Part model, mm, in its own coordinate system. A direction names the side the tool comes from. Give positions to 0.01 mm unless a question says otherwise; leave off trailing zeros. Order: outer loops, then holes, each group sorted by start corner. A loop starts at its lowest first (then second) coordinate and runs counter-clockwise, first axis right, second up.
1. Probe line 1 (X direction, y = -17.25, z = 0); line 2 (Z direction, x = -14.5, y = -19.25); line 3 (Z direction, x = -17, y = -25). List the from-to ranges inside material, lowest first.
2. Slice it at C-C on y = -12.5. List the corners of the cut face in (x, z).
3. Which spindle directions (+Z, -Z, +X, -X, +Y, -Y) get a long thin tool onto all of the face, cutting with end or side? Do faces 4 (the cylindrical face through (-19.62, -15.42, 2.95)), 5 (the flat face through (-14, -8.753, 4)). Say none if no direction does.
4. Mould opens along Y. For faces 1 (the cylindrical face through (-17.355, -15.705, 5.207)), 2 (the flat face through (-20, -21.753, 1)), 3 (the flat face through (-18, -33.753, -3)) say: +Y half, -Y half, draft (parallel to the pull), parting line (faces both ways), or undercut.
5. Drop flat-ended pins along their axis: pin 1 Ø2 at (x, z) = (-20, 0) entering from +Y; pin 2 Ø4 at (x, y) = (-20.5, -15) entering from +Z; pin 3 Ø4 at (x, y) = (-12, -12) entering from +Z; pin 4 Ø5 at (x, y) = (-16.92, -28.75) entering from +Z. Give the stop position or say it passes through.
6. Slice it at D-D on y = -16.25. List the corners of the cut face in (x, z).
7. Slice it at A-A on y = -30. List the corners of the cut face in (x, z).
8. Slice it at B-B on x = -15.25. Give the number of separate pieces and of enclosed holes in the cut face, and give its area (3 significant figures).
from build123d import *

# Parameters (mm, degrees)
WYTNIJ_WYCI_GNI_CIE1_DEPTH      = 42.958230131
WYTNIJ_WYCI_GNI_CIE1_DEPTH_BACK = 42.958230131
SZKIC2_R                        = 2
SFAZOWANIE1_SIZE                = 0.5
ZAOKR_GLENIE1_R                 = 0.5
SFAZOWANIE2_SIZE                = 0.5


with BuildPart() as part:
    # Szkic1 → Obrót1 (revolve)
    with BuildSketch(Plane.XY, mode=Mode.PRIVATE) as obr_t1_sk:
        Polygon((-20.921239747, -8.753034896), (-23.921239747, -8.753034896), (-23.921239747, -33.753034896), (-19.421239747, -33.753034896), (-19.421239747, -21.753034896), (-20.921239747, -21.753034896), align=None)
    revolve(obr_t1_sk.sketch.rotate(Axis((-16.921239747, -33.753034896, 0), (0, 1, 0)), 270), axis=Axis((-16.921239747, -33.753034896, 0), (0, 1, 0)))

    # Szkic2 → Wytnij-wyciągnięcie1 (cut, two sides: drawn at the far end of the back side and taken through both)
    with BuildSketch(Plane.XY.offset(-WYTNIJ_WYCI_GNI_CIE1_DEPTH_BACK)):
        with Locations((-16.921239747, -13.753034896)):
            Circle(SZKIC2_R)
        with Locations((-16.921239747, -28.753034896)):
            Circle(SZKIC2_R)
    extrude(amount=WYTNIJ_WYCI_GNI_CIE1_DEPTH + WYTNIJ_WYCI_GNI_CIE1_DEPTH_BACK, mode=Mode.SUBTRACT)

    # Sfazowanie1
    sfazowanie1_edges = [part.edges().sort_by_distance(p)[0] for p in [
        (-16.921239747, -33.753034896, 2.5),
        (-16.921239747, -33.753034896, 7),
        (-16.921239747, -8.753034896, 7),
        (-16.921239747, -8.753034896, 4),
    ]]
    chamfer(sfazowanie1_edges, length=SFAZOWANIE1_SIZE)

    # Zaokrąglenie1
    zaokr_glenie1_edges = [part.edges().sort_by_distance(p)[0] for p in [
        (-16.921239747, -33.753034896, 6.5),
        (-16.921239747, -9.253034896, 7),
        (-16.921239747, -33.253034896, 7),
        (-16.921239747, -8.753034896, 6.5),
    ]]
    fillet(zaokr_glenie1_edges, radius=ZAOKR_GLENIE1_R)

    # Sfazowanie2
    sfazowanie2_edges = [part.edges().sort_by_distance(p)[0] for p in [
        (-16.921239747, -21.753034896, 2.5),
    ]]
    chamfer(sfazowanie2_edges, length=SFAZOWANIE2_SIZE)


solid = part.part
Data:
1. line 1: x = -23.92 to -20.92, -12.92 to -9.92
1. line 2: z = -6.57 to -3.18, 3.18 to 6.57
1. line 3: z = -7 to -2.5, 2.5 to 7
2. outline: (-18.48, -6.82) - (-18.48, -3.68) arc R4 cw to (-18.48, 3.68) - (-18.48, 6.82) arc R7 ccw to start; (-15.36, -6.82) arc R7 ccw to (-15.36, 6.82) - (-15.36, 3.68) arc R4 cw to (-15.36, -3.68) - close
3. face 4: +Y
3. face 5: +Z, -Z, +X, -X, +Y
4. face 1: undercut
4. face 2: +Y half
4. face 3: -Y half
5. pin 1: stops at y = -9.17
5. pin 2: stops at z = 6.82
5. pin 3: stops at z = 6.36
5. pin 4: stops at z = 7
6. outline: circle Ø14 at (-16.92, 0); hole circle Ø8 at (-16.92, 0)
7. outline: (-18.48, -6.82) - (-18.48, -1.95) arc R2.5 cw to (-18.48, 1.95) - (-18.48, 6.82) arc R7 ccw to start; (-15.36, -6.82) arc R7 ccw to (-15.36, 6.82) - (-15.36, 1.95) arc R2.5 cw to (-15.36, -1.95) - close
8. separate pieces: 6
8. enclosed holes: 0
8. area: 164 mm2
